Design review of the part built by this model. Coordinates are the model's own, in mm. A direction names the side the tool comes from. Round coordinates to 2 decimals unless told otherwise and drop trailing zeros. Order: outer loops, then holes, each group sorted by start corner. A loop starts at its lowest first (then second) coordinate and runs counter-clockwise, first axis right, second up. Notation, with made-up numbers: M -39,49.25 L 19,49.25 A23 ccw 19,76.25 Z; hole C 7,70.25 d5. An arc over 180 degrees is marked long. Write each question's results on one line, items separated by ' | '. Start each with the question number.
Item 1: Clearance check with flat-ended pins moving along their axes: pin 1 (2 mm diameter, centred on y = 10, z = 12, fed in from +X); pin 2 (4 mm diameter, centred on x = 11, z = 25.5, fed in from +Y). State where each tip first meets the part, or that it passes through.
Item 2: Machinability: for faces 1 (the flat face through (2.5, 9, 0)), 2 (the flat face through (-28, 12, 0)), which of the approach directions +Z, -Z, +X, -X, +Y, -Y give a long, thin tool a straight path to every point of the face, cutting with its end or side? Answer none if there is none.
Item 3: Wall thickness on line 1 (X direction, y = 10.75, z = 30); line 2 (Y direction, x = 28.5, z = -11): over which ranges is each line inside the solid? List them lowest first. Write a range as [from, to].
Item 4: Take a section at B-B, the plane x = 19.5. Write out the cut boundary in (y, z).
Item 5: Take a section at A-A, the plane z = 1.5. Write out the cut boundary in (x, y), plus the area to 4 significant figures.
Item 6: Take a section at C-C, the plane y = 9.25. Write out the cut boundary in (x, z), plus the area to 3 significant figures.
```python
from build123d import *

# Parameters (mm, degrees)
SKETCH_1_W               = 115
SKETCH_1_H               = 65
EXTRUDE_1_DEPTH          = 12
CUT_EXTRUDE_1_DEPTH      = 68.130469982
CUT_EXTRUDE_1_DEPTH_BACK = 68.130469982
SKETCH_3_W               = 55
SKETCH_3_H               = 5


with BuildPart() as part:
    # 스케치1 → 보스-돌출1 (new body)
    with BuildSketch(Plane(origin=(0, 0, 0), x_dir=(1, 0, 0), z_dir=(0, 1, 0))):
        Rectangle(SKETCH_1_W, SKETCH_1_H)
    extrude(amount=EXTRUDE_1_DEPTH)

    # 스케치3 → 컷-돌출1 (cut, two sides: drawn at the far end of the back side and taken through both)
    with BuildSketch(Plane.XY.offset(-CUT_EXTRUDE_1_DEPTH_BACK)):
        with Locations((30, 9.5)):
            Rectangle(SKETCH_3_W, SKETCH_3_H)
    extrude(amount=CUT_EXTRUDE_1_DEPTH + CUT_EXTRUDE_1_DEPTH_BACK, mode=Mode.SUBTRACT)


solid = part.part
```
Results list:
1) pin 1: x = 2.5 | pin 2: y = 7
2) face 1: +Z, -Z, +X, +Y | face 2: +Z, -Z, +X, -X, +Y
3) line 1: [-57.5, 2.5] | line 2: [0, 7]
4) outline: M 0,-32.5 L 7,-32.5 L 7,32.5 L 0,32.5 Z
5) outline: M -57.5,0 L 57.5,0 L 57.5,7 L 2.5,7 L 2.5,12 L -57.5,12 Z | area: 1,105 mm²
6) outline: M -57.5,-32.5 L 2.5,-32.5 L 2.5,32.5 L -57.5,32.5 Z | area: 3,900 mm²
